Can you work these out from the model? Positions are in its coordinate system, mm. Round coordinates to 2 decimals unless told otherwise and drop trailing zeros. Loops run counter-clockwise (first coordinate to the right, second up) from the corner with the lowest first, then second, coordinate; pieces in that order, holes last. Notation, with made-up numbers: M -39,79.25 L 2,79.25 A10 cw 2,90.25 Z; hole C 51,27 d5. An arc over 180 degrees is marked long. Return JSON: item names as keys, results as strings.
```python
from build123d import *

# Parameters (mm, degrees)
BOSS_EXTRUDE1_DEPTH = 5
SKETCH2_R           = 2
CUT_EXTRUDE1_DEPTH  = 5


with BuildPart() as part:
    # Sketch1 → Boss-Extrude1 (new body)
    with BuildSketch(Plane(origin=(0, 0, 0), x_dir=(1, 0, 0), z_dir=(0, 1, 0))):
        Polygon((9.270509831, -12.759762125), (15, -4.873795443), (15, 4.873795443), (9.270509831, 12.759762125), (0, 15.771933364), (-9.270509831, 12.759762125), (-15, 4.873795443), (-15, -4.873795443), (-9.270509831, -12.759762125), (0, -15.771933364), align=None)
    extrude(amount=BOSS_EXTRUDE1_DEPTH)

    # Sketch2 → Cut-Extrude1 (cut)
    with BuildSketch(Plane(origin=(0, 5, 0), x_dir=(1, 0, 0), z_dir=(0, 1, 0))):
        Circle(SKETCH2_R)
        with Locations((9.303695435, 6.759530401)):
            Circle(SKETCH2_R)
    extrude(amount=-CUT_EXTRUDE1_DEPTH, mode=Mode.SUBTRACT)


solid = part.part
```
Q1. Suppose I cut it at B-B, the plane y = 3.3. Please give me the cut outline in (x, z).
Results:
{"outline": "M -15,-4.87 L -9.27,-12.76 L 0,-15.77 L 9.27,-12.76 L 15,-4.87 L 15,4.87 L 9.27,12.76 L 0,15.77 L -9.27,12.76 L -15,4.87 Z; hole C 0,0 d4; hole C 9.3,-6.76 d4"}
Q2. I'm going to push flat-ended pins straight in: pin 1 Ø2 at (y, z) = (1, 6) entering from +X; pin 2 Ø2.5 at (x, z) = (9.3, -6.76) entering from +Y; pin 3 Ø2 at (x, y) = (-11, 1.5) entering from -Z; pin 4 Ø3 at (y, z) = (2, 12) entering from +X. Where does each tip first touch, or does it pass through?
Results:
{"pin 1": "stops at x = 14.91", "pin 2": "passes through", "pin 3": "stops at z = -11.76", "pin 4": "stops at x = 10.91"}
Q3. Suppose I cut it at D-D, the plane z = 14. Please give me the cut outline in (x, y), plus the area to 3 significant figures.
Results:
{"outline": "M -5.45,0 L 5.45,0 L 5.45,5 L -5.45,5 Z", "area": "54.5 mm2"}
Q4. Suppose I cut it at A-A, the plane z = 0. Please give me the cut outline in (x, y), plus the area to 3 significant figures.
Results:
{"outline": "M -15,0 L -2,0 L -2,5 L -15,5 Z; M 2,0 L 15,0 L 15,5 L 2,5 Z", "area": "130 mm2"}
Q5. Suppose I cut it at C-C, the plane x = -11. Please give me the cut outline in (y, z).
Results:
{"outline": "M 0,-10.38 L 5,-10.38 L 5,10.38 L 0,10.38 Z"}
Q6. If I drill on line 1 along X through (y, z) = (2.4, 0); line 2 along X through (y, z) = (2.2, -5.5); line 3 along Z through (x, y) = (10, 4.85), over which ranges is the centre line in solid material (lowest first)?
Results:
{"line 1": "x = -15 to -2, 2 to 15", "line 2": "x = -14.55 to 7.75, 10.86 to 14.55", "line 3": "z = -11.76 to -8.63, -4.88 to 11.76"}
Q7. Thinking about a two-plate mould opening in X: for faces 1 (the cylindrical face through (0, 3, 2)), 2 (the flat face through (-12, 2, 9)), 3 (the flat face through (4.7, 2.465, -14.245)), which applies, pulls with the +X half, pulls with the -X half, needs draft (parallel to the pull), parting line crosses it, or undercut?
Results:
{"face 1": "undercut", "face 2": "pulls with the -X half", "face 3": "pulls with the +X half"}
